Could you check a few things on this drawing? It's one solid part, dimensions in mm from its lowest x, y, z. A direction names the side the tool comes from. Give positions to 0.01 mm unless a question says otherwise; leave off trailing zeros. Order: outer loops, then holes, each group sorted by start corner. A loop starts at its lowest first (then second) coordinate and runs counter-clockwise, first axis right, second up.
Item 1: I'm going to push flat-ended pins straight in: pin 1 Ø8 at (x, z) = (16, 137.5) entering from -Y; pin 2 Ø3 at (y, z) = (40.5, 59.5) entering from -X. Where does each tip first touch, or does it pass through?
Item 2: I want a section at A-A, the plane z = 100. Write out the boundary of the cut face in (x, y).
Item 3: Which directions (+Z, -Z, +X, -X, +Y, -Y) give clear straight access to the entire face, cutting with the end or side of a thin tool? Please do the marked faces 1, 2 and 3.
Item 4: If I drill on line 1 along Z through (x, y) = (50, 25); line 2 along Y through (x, z) = (41, 189); line 3 along X through (y, z) = (17.5, 31), over which ranges is the centre line in solid material (lowest first)?
Item 5: I want a section at D-D, the plane z = 170. Write out the boundary of the cut face in (x, y).
Item 6: I want a section at C-C, the plane y = 34. Write out the boundary of the cut face in (x, z), then the cut area to 3 significant figures.
Item 7: I want a section at B-B, the plane x = 50. Write out the boundary of the cut face in (y, z).
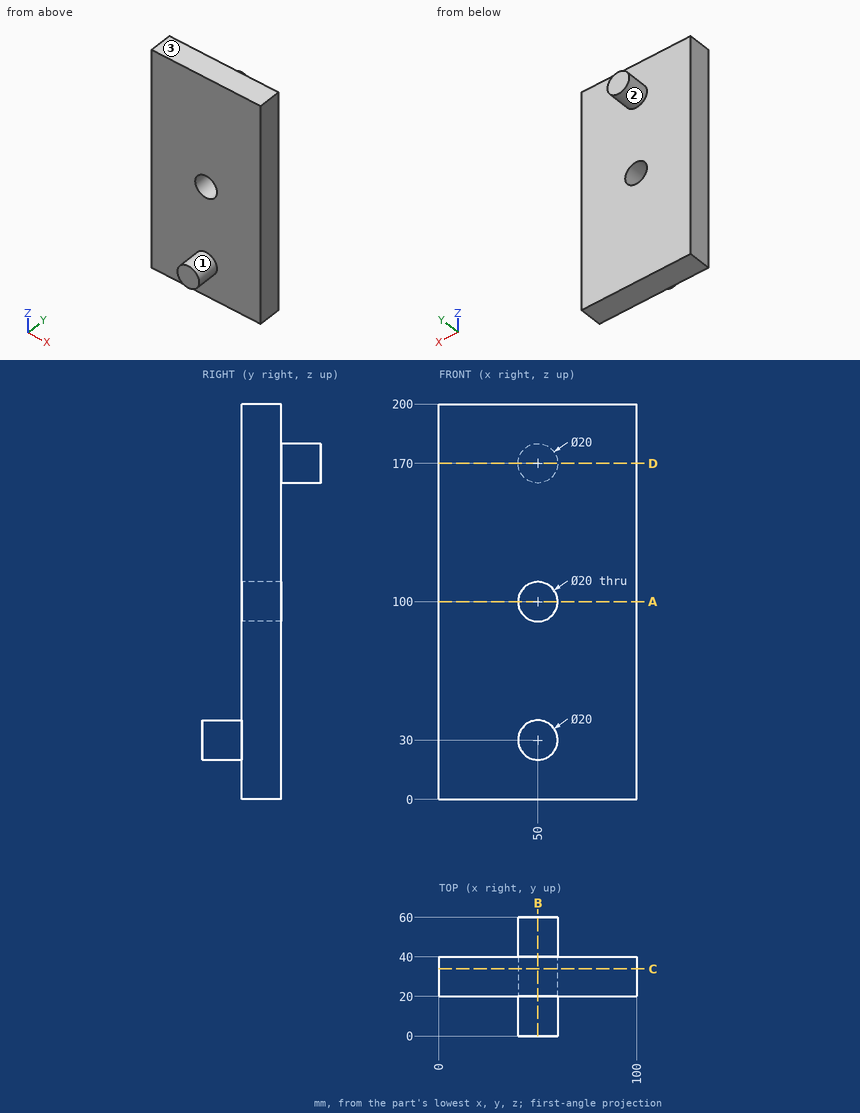
Results list:
1. pin 1: stops at y = 20
1. pin 2: stops at x = 0
2. outline: (0, 20) - (40, 20) - (40, 40) - (0, 40) - close; (60, 20) - (100, 20) - (100, 40) - (60, 40) - close
3. face 1: -Y
3. face 2: +Y
3. face 3: +Z, +X, -X, +Y, -Y
4. line 1: z = 0 to 90, 110 to 200
4. line 2: y = 20 to 40
4. line 3: x = 40.05 to 59.95
5. outline: (0, 20) - (100, 20) - (100, 40) - (60, 40) - (60, 60) - (40, 60) - (40, 40) - (0, 40) - close
6. outline: (0, 0) - (100, 0) - (100, 200) - (0, 200) - close; hole circle Ø20 at (50, 100)
6. area: 19,700 mm2
7. outline: (0, 20) - (20, 20) - (20, 0) - (40, 0) - (40, 90) - (20, 90) - (20, 40) - (0, 40) - close; (20, 110) - (40, 110) - (40, 160) - (60, 160) - (60, 180) - (40, 180) - (40, 200) - (20, 200) - close
